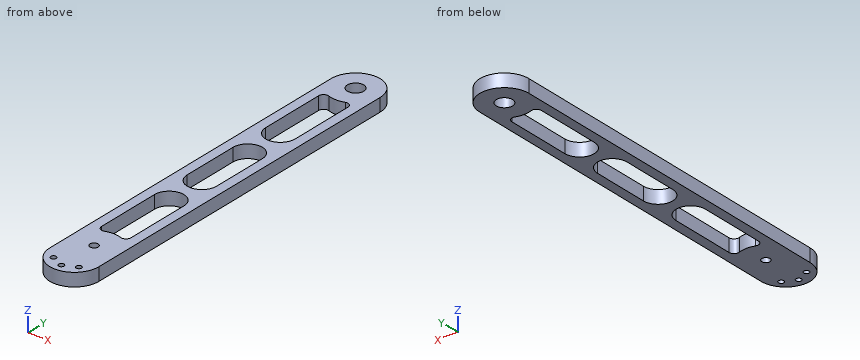
from build123d import *

# Parameters (mm, degrees)
SKETCH_1_R      = 5.025
SKETCH_1_R_2    = 2.525
EXTRUDE_1_DEPTH = 8
SKETCH_2_R      = 1.65
EXTRUDE_2_DEPTH = 8


with BuildPart() as part:
    # 草图1 → 凸台-拉伸1 (new body)
    with BuildSketch(Plane.XY):
        with BuildLine():
            Line((-15, 0), (-15, -200))
            ThreePointArc((-15, -200), (0, -215), (15, -200))
            Line((15, -200), (15, 0))
            ThreePointArc((15, 0), (0, 15), (-15, 0))
        make_face()
        Circle(SKETCH_1_R, mode=Mode.SUBTRACT)
        with Locations((0, -200)):
            Circle(SKETCH_1_R_2, mode=Mode.SUBTRACT)
        with BuildLine():
            Line((-9, -16.970562748), (-9, -57.5))
            ThreePointArc((-9, -57.5), (0, -66.5), (9, -57.5))
            Line((9, -57.5), (9, -16.970562748))
            ThreePointArc((9, -16.970562748), (7.732050808, -14.521073006), (5, -14.142135624))
            ThreePointArc((5, -14.142135624), (0, -15), (-5, -14.142135624))
            ThreePointArc((-5, -14.142135624), (-7.732050808, -14.521073006), (-9, -16.970562748))
        make_face(mode=Mode.SUBTRACT)
        with BuildLine():
            Line((9, -82.5), (9, -117.5))
            ThreePointArc((9, -117.5), (0, -126.5), (-9, -117.5))
            Line((-9, -117.5), (-9, -82.5))
            ThreePointArc((-9, -82.5), (0, -73.5), (9, -82.5))
        make_face(mode=Mode.SUBTRACT)
        with BuildLine():
            Line((-9, -183.029437252), (-9, -142.5))
            ThreePointArc((-9, -142.5), (0, -133.5), (9, -142.5))
            Line((9, -142.5), (9, -183.029437252))
            ThreePointArc((9, -183.029437252), (7.732050808, -185.478926994), (5, -185.857864376))
            ThreePointArc((5, -185.857864376), (0, -185), (-5, -185.857864376))
            ThreePointArc((-5, -185.857864376), (-7.732050808, -185.478926994), (-9, -183.029437252))
        make_face(mode=Mode.SUBTRACT)
    extrude(amount=EXTRUDE_1_DEPTH)

    # 草图2 → 凸台-拉伸2 (add, through all)
    with BuildSketch(Plane.XY):
        with BuildLine():
            Line((-15, -200), (-15, -215))
            ThreePointArc((-15, -215), (0, -230), (15, -215))
            Line((15, -215), (15, -200))
            ThreePointArc((15, -200), (0, -215), (-15, -200))
        make_face()
        with Locations((0, -225)):
            Circle(SKETCH_2_R, mode=Mode.SUBTRACT)
        with Locations((-7.756707253, -221.311378027)):
            Circle(SKETCH_2_R, mode=Mode.SUBTRACT)
        with Locations((7.756707253, -221.311378027)):
            Circle(SKETCH_2_R, mode=Mode.SUBTRACT)
    extrude(amount=EXTRUDE_2_DEPTH)


solid = part.part
Work out the finished part from the listing and answer in its coordinate system (mm). Give positions to 0.01 mm unless a question says otherwise; leave off trailing zeros. Write each loop counter-clockwise with the first axis right and the second up, starting at its lowest first coordinate (ties: lowest second). Pieces come first, ordered by that corner, then holes. Notation, with made-up numbers: (1.5, 79) - (14.5, 79) arc R28 cw to (14.5, 111) - close; hole circle Ø5 at (16, 50.5). An arc over 180 degrees is marked (long way). One line per item, written item: value. Start each with the question number.
1. Given pin 1 (3 mm diameter, centred on x = 10.5, z = 1, fed in from +Y); pin 2 (4 mm diameter, centred on x = 0, y = -225, fed in from -Z); pin 3 (3 mm diameter, centred on x = 10, z = 4.5, fed in from +Y); pin 4 (1.5 mm diameter, centred on x = -11, z = 3, fed in from -Y), each flat-ended and moving along its own axis, determine where each tip first touches the part or whether it passes through.
2. Find section B-B (y = -200). Write down the section's boundary in (x, z) (3 decimals).
3. Find section A-A (y = -175). Write down the section's boundary in (x, z), then the cut area to 3 significant figures.
4. Consider probe 1 along X at (y, z) = (-31, 6.5); probe 2 along X at (y, z) = (-125, 1.5); probe 3 along Y at (x, z) = (-7, 4). Determine where each line is inside the solid, lowest interval first.
5. Find section C-C (z = 3). State how many separate pieces and enclosed holes the cut face has, then the cut area to 3 significant figures.
6. Find section D-D (x = 11.5). Write down the section's boundary in (y, z), then the cut area to 3 significant figures.
Geometry results:
1. pin 1: y = 12
1. pin 2: z = 0
1. pin 3: y = 12.36
1. pin 4: y = -225.95
2. outline: (-15, 0) - (-2.525, 0) - (-2.525, 8) - (-15, 8) - close; (2.525, 0) - (15, 0) - (15, 8) - (2.525, 8) - close
3. outline: (-15, 0) - (-9, 0) - (-9, 8) - (-15, 8) - close; (9, 0) - (15, 0) - (15, 8) - (9, 8) - close
3. area: 96.0 mm2
4. probe 1: -15 to -9, 9 to 15
4. probe 2: -15 to -4.97, 4.97 to 15
4. probe 3: -228.27 to -222.78, -219.85 to -185.86, -136.84 to -123.16, -76.84 to -63.16, -14.14 to 13.27
5. separate pieces: 1
5. enclosed holes: 8
5. area: 4,350 mm2
6. outline: (-224.63, 0) - (9.63, 0) - (9.63, 8) - (-224.63, 8) - close
6. area: 1,870 mm2
